The figure shows three views and two pictorial views of one solid part (mm, origin at its lowest corner). Answer the questions. Round coordinates to 2 decimals unless told otherwise and drop trailing zeros. Order: outer loops, then holes, each group sorted by start corner. A loop starts at its lowest first (then second) coordinate and runs counter-clockwise, first axis right, second up. Notation, with made-up numbers: (0, 54) -> (29, 54) arc R21 ccw to (29, 88) -> close; hole circle Ø3 at (1, 22). An arc over 180 degrees is marked (long way). Answer as a JSON object with one key per item and string values. Group by question number.
Item 1: Section A-A, the plane x = 133 is taken. Write down the section's boundary in (y, z).
Item 2: Consider probe 1 along Y at (x, z) = (136.5, 1.75); probe 2 along Y at (x, z) = (117.5, 2.35); probe 3 along X at (y, z) = (82.5, 1.35). Determine where each line is inside the solid, lowest interval first. Write a range as from..to.
Item 3: Section C-C, the plane z = 1.1 is taken. Count the separate pieces of the cut face and the enclosed holes in it, plus the area to 3 significant figures.
Item 4: Section B-B, the plane y = 69 is taken. Write down the section's boundary in (x, z), plus the area to 3 significant figures.
Item 5: Given P1, Ø3, axis at x = 172.5, y = 59.5, coming from the -Z side, flat-ended and moving along its own axis, determine where the tip first touches the part or whether it passes through.
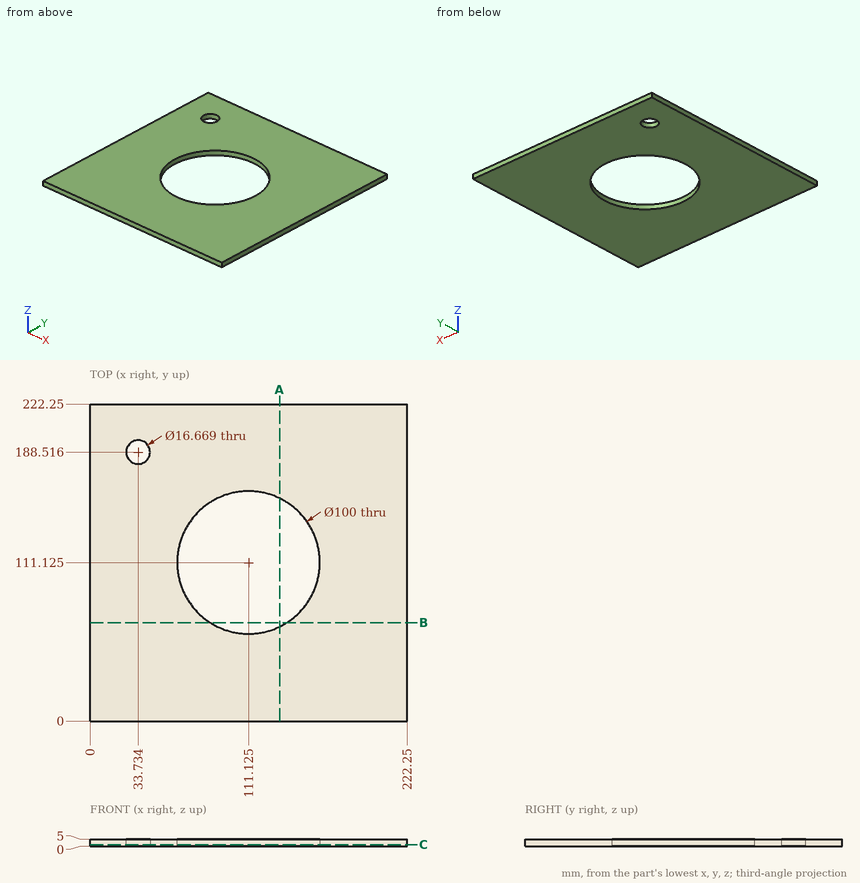
Values found:
{
 "1": {"outline": "(0, 0) -> (66.16, 0) -> (66.16, 5) -> (0, 5) -> close; (156.09, 0) -> (222.25, 0) -> (222.25, 5) -> (156.09, 5) -> close"},
 "2": {"probe 1": "0..68.04, 154.21..222.25", "probe 2": "0..61.53, 160.72..222.25", "probe 3": "0..70.13, 152.12..222.25"},
 "3": {"separate pieces": "1", "enclosed holes": "2", "area": "41,300 mm2"},
 "4": {"outline": "(0, 0) -> (84.19, 0) -> (84.19, 5) -> (0, 5) -> close; (138.06, 0) -> (222.25, 0) -> (222.25, 5) -> (138.06, 5) -> close", "area": "842 mm2"},
 "5": {"P1": "z = 0"}
}
